```python
from build123d import *

# Parameters (mm, degrees)
SKETCH024_W         = 210
SKETCH024_H         = 140
PAD014_DEPTH        = 15
SKETCH025_R         = 7.6
POCKET006_DEPTH     = 35
HOLE004_D           = 4.2
HOLE004_DEPTH       = 25
HOLE004_CSINK_D     = 11.2
HOLE004_CSINK_ANGLE = 90
SKETCH029_R         = 2.75
HOLE007_DEPTH       = 40
HOLE007_TIPS_R      = 2.75


with BuildPart() as part:
    # Sketch024 → Pad014 (new body)
    with BuildSketch(Plane.YZ):
        with Locations((0, -5)):
            Rectangle(SKETCH024_W, SKETCH024_H)
    extrude(amount=-PAD014_DEPTH)

    # Sketch025 → Pocket006 (cut)
    with BuildSketch(Plane.YZ):
        Circle(SKETCH025_R)
    extrude(amount=-POCKET006_DEPTH, mode=Mode.SUBTRACT)

    # Hole004
    with Locations(Plane(origin=(-15, 0, 0), x_dir=(0, 1, 0), z_dir=(-1, 0, 0))):
        with Locations((-95, 65), (-75, 65), (95, 65), (75, 65), (-87.5, -57.5), (87.5, -57.5)):
            CounterSinkHole(HOLE004_D / 2, HOLE004_CSINK_D / 2, depth=HOLE004_DEPTH, counter_sink_angle=HOLE004_CSINK_ANGLE)

    # Sketch029 → Hole007 (cut)
    with BuildSketch(Plane.XY.offset(65)):
        with Locations((-7.5, -97.5)):
            Circle(SKETCH029_R)
        with Locations((-7.5, 97.5)):
            Circle(SKETCH029_R)
    extrude(amount=-HOLE007_DEPTH, mode=Mode.SUBTRACT)

    # Hole007 tips → Hole007 tip 1 section 0
    with BuildSketch(Plane.XY.offset(25), mode=Mode.PRIVATE) as hole007_tip_1_s0:
        with Locations((-7.5, -97.5)):
            Circle(HOLE007_TIPS_R)
    loft([hole007_tip_1_s0.sketch, Vertex(-7.5, -97.5, 23.347633)], mode=Mode.SUBTRACT)

    # Hole007 tips → Hole007 tip 2 section 0
    with BuildSketch(Plane.XY.offset(25), mode=Mode.PRIVATE) as hole007_tip_2_s0:
        with Locations((-7.5, 97.5)):
            Circle(HOLE007_TIPS_R)
    loft([hole007_tip_2_s0.sketch, Vertex(-7.5, 97.5, 23.347633)], mode=Mode.SUBTRACT)


solid = part.part
```
Design review of the part built by this model. Coordinates are the model's own, in mm. A direction names the side the tool comes from. Round coordinates to 2 decimals unless told otherwise and drop trailing zeros. Write each loop counter-clockwise with the first axis right and the second up, starting at its lowest first coordinate (ties: lowest second). Pieces come first, ordered by that corner, then holes.
Item 1: We need section B-B on z = 0. Write out the cut boundary in (x, y).
Item 2: Clearance check with flat-ended pins moving along their axes: pin 1 Ø5.5 at (y, z) = (-95, -65) entering from -X; pin 2 Ø6.5 at (y, z) = (-75, -65) entering from -X; pin 3 Ø3.5 at (x, y) = (-7.5, -97.5) entering from +Z. State where each tip first meets the part, or that it passes through.
Item 3: The part is to be moulded in two halves that separate along Z. For faces 3 (the flat face through (-7, -105, -6)), 4 (the flat face through (-7, -1, 65)), 5 (the conical face through (-11.67, 92.835, -65.682)), say which applies: +Z half, -Z half, draft (parallel to the pull), parting line (faces both ways), or undercut.
Item 4: We need section C-C on y = 0. Write out the cut boundary in (x, z).
Item 5: For probe 1 along Y at (x, z) = (-4.25, -65); probe 2 along Z at (x, y) = (-3.75, 87.5); probe 3 along Z at (x, y) = (-3, -75), list the stretches that pass through material, from the lowest coordinate up.
Item 6: For faces 1 (the conical face through (-11.67, -87.008, 59.716)), 2 (the cylindrical face through (-8.096, -100.185, 45.28)), list the 3-axis set-ups (+Z, -Z, +X, -X, +Y, -Y) from which the entire face can be reached by the end or side of a thin tool; tool diameter is ignored.
Item 7: We need section A-A on z = 57.5. Write out the cut boundary in (x, y).
Returned:
1. outline: (-15, -105) - (0, -105) - (0, -7.6) - (-15, -7.6) - close; (-15, 7.6) - (0, 7.6) - (0, 105) - (-15, 105) - close
2. pin 1: stops at x = -12.15
2. pin 2: stops at x = -12.65
2. pin 3: stops at z = 24.4
3. face 3: draft
3. face 4: +Z half
3. face 5: undercut
4. outline: (-15, -75) - (0, -75) - (0, -7.6) - (-15, -7.6) - close; (-15, 7.6) - (0, 7.6) - (0, 65) - (-15, 65) - close
5. probe 1: y = -105 to -97.1, -92.9 to -77.1, -72.9 to 72.9, 77.1 to 92.9, 97.1 to 105
5. probe 2: z = -75 to 55.4, 59.6 to 65
5. probe 3: z = -75 to -67.1, -62.9 to 65
6. face 1: -X
6. face 2: +Z
7. outline: (-15, -105) - (0, -105) - (0, -89.6) - (-11.5, -89.6) - (-15, -93.1) - close; (-15, -81.9) - (-11.5, -85.4) - (0, -85.4) - (0, 85.4) - (-11.5, 85.4) - (-15, 81.9) - close; (-15, 93.1) - (-11.5, 89.6) - (0, 89.6) - (0, 105) - (-15, 105) - close; hole circle Ø5.5 at (-7.5, -97.5); hole circle Ø5.5 at (-7.5, 97.5)
